from build123d import *

# Parameters (mm, degrees)
F1_DEPTH       = 120.65
F2_R           = 1.524
F4_D           = 20.6375
F4_CBORE_D     = 30.1752
F4_CBORE_DEPTH = 28.448
F5_W           = 63.5
F5_H           = 241.3
F6_DEPTH       = 6.35
F8_D           = 13.49248
F8_DEPTH       = 41.2172727273
F8_TIP         = 4.0535499425


# Not quite as in the source:
# - a length typed as a fraction of an inch, garbled in the dataset ("3 / 203.2 mm" for 3/8 in), is restored


with BuildPart() as f1:
    # F0 (on Top) → F1 (new body, symmetric)
    with BuildSketch(Plane.XY):
        Polygon((82.55, 44.45), (-82.55, 44.45), (-82.55, 31.75), (-44.45, 31.75), (-44.45, -31.75), (-82.55, -31.75), (-82.55, -44.45), (82.55, -44.45), align=None)
    extrude(amount=F1_DEPTH, both=True)

    # F2
    f2_edges = [f1.edges().sort_by_distance(p)[0] for p in [
        (-44.45, 31.75, 0),
        (-44.45, -31.75, 0),
    ]]
    fillet(f2_edges, radius=F2_R)

    # F4 (through all)
    with Locations(Plane.YZ.offset(82.55)):
        with Locations((0, 63.5), (0, -63.5)):
            CounterBoreHole(F4_D / 2, F4_CBORE_D / 2, F4_CBORE_DEPTH)

    # F5 (on face) → F6 (cut)
    with BuildSketch(Plane.XZ.offset(44.45)):
        with Locations((50.8, 0)):
            Rectangle(F5_W, F5_H)
    extrude(amount=-F6_DEPTH, mode=Mode.SUBTRACT)

    # F8
    with Locations(Plane.XZ.offset(38.1)):
        with Locations((50.8, 95.25), (50.8, 0), (50.8, -95.25)):
            Hole(F8_D / 2, depth=F8_DEPTH)
            with Locations((0, 0, -(F8_DEPTH + F8_TIP / 2))):  # 118° drill point
                Cone(0, F8_D / 2, F8_TIP, mode=Mode.SUBTRACT)


solid = f1.part
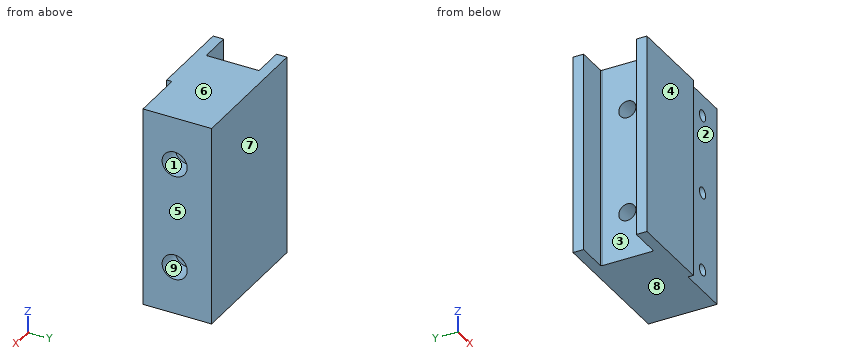
Could you check a few things on this model? Use its own coordinates, in mm. Face numbers are marked on the shaded views. A direction names the side the tool comes from. Round coordinates to 2 decimals unless told otherwise and drop trailing zeros. Order: outer loops, then holes, each group sorted by start corner. A loop starts at its lowest first (then second) coordinate and runs counter-clockwise, first axis right, second up.
(1) Imagine slicing it at A-A (y = 0). Write out the boundary of the cut face in (x, z), plus the area to 3 significant figures.
Response values:
outline: (-44.45, -120.65) - (82.55, -120.65) - (82.55, -78.59) - (54.1, -78.59) - (54.1, -73.82) - (-44.45, -73.82) - close; (-44.45, -53.18) - (54.1, -53.18) - (54.1, -48.41) - (82.55, -48.41) - (82.55, 48.41) - (54.1, 48.41) - (54.1, 53.18) - (-44.45, 53.18) - close; (-44.45, 73.82) - (54.1, 73.82) - (54.1, 78.59) - (82.55, 78.59) - (82.55, 120.65) - (-44.45, 120.65) - close; hole circle Ø13.49 at (50.8, -95.25); hole circle Ø13.49 at (50.8, 0); hole circle Ø13.49 at (50.8, 95.25)
area: 24,400 mm2
(2) I'm going to push flat-ended pins straight in: pin 1 (9 mm diameter, centred on y = 5.5, z = -59, fed in from +X); pin 2 (3 mm diameter, centred on y = -14.5, z = -48.5, fed in from -X); pin 3 (8 mm diameter, centred on x = 50.8, z = 95.25, fed in from -Y); pin 4 (24 mm diameter, centred on y = -2, z = 71, fed in from +X). Where does each tip first touch, or does it pass through?
Response values:
pin 1: stops at x = 54.1
pin 2: stops at x = -44.45
pin 3: stops at y = 4.77
pin 4: stops at x = 82.55
(3) Which directions (+Z, -Z, +X, -X, +Y, -Y) give clear straight access to the entire face, cutting with the end or side of a thin tool? Please do the marked faces 1, 2, 3, 4 and 5.
Response values:
face 1: +X
face 2: +Z, -Z, +X, -Y
face 3: +Z, -Z, -X
face 4: +Z, -Z, +X, -X, -Y
face 5: +Z, -Z, +X, +Y, -Y
(4) Please list where these lines run through material, in increasing order: line 1 along Z through (x, y) = (68, 0); line 2 along Z through (x, y) = (32, 0); line 3 along Z through (x, y) = (50.8, -24.5).
Response values:
line 1: z = -120.65 to -78.59, -48.41 to 48.41, 78.59 to 120.65
line 2: z = -120.65 to -73.82, -53.18 to 53.18, 73.82 to 120.65
line 3: z = -120.65 to -102, -88.5 to -6.75, 6.75 to 88.5, 102 to 120.65
(5) Imagine slicing it at B-B (x = -54). Write out the boundary of the cut face in (y, z), plus the area to 3 significant figures.
Response values:
outline: (-44.45, -120.65) - (-31.75, -120.65) - (-31.75, 120.65) - (-44.45, 120.65) - close; (31.75, -120.65) - (44.45, -120.65) - (44.45, 120.65) - (31.75, 120.65) - close
area: 6,130 mm2
(6) Imagine slicing it at D-D (x = -0.5). Write out the boundary of the cut face in (y, z).
Response values:
outline: (-44.45, -120.65) - (44.45, -120.65) - (44.45, 120.65) - (-44.45, 120.65) - close; hole circle Ø20.64 at (0, -63.5); hole circle Ø20.64 at (0, 63.5)
(7) Imagine slicing it at C-C (z = 63.5). Write out the boundary of the cut face in (x, y), plus the area to 3 significant figures.
Response values:
outline: (-82.55, -44.45) - (19.05, -44.45) - (19.05, -38.1) - (82.55, -38.1) - (82.55, -15.09) - (54.1, -15.09) - (54.1, -10.32) - (-44.45, -10.32) - (-44.45, -30.23) arc R1.52 cw to (-45.97, -31.75) - (-82.55, -31.75) - close; (-82.55, 31.75) - (-45.97, 31.75) arc R1.52 cw to (-44.45, 30.23) - (-44.45, 10.32) - (54.1, 10.32) - (54.1, 15.09) - (82.55, 15.09) - (82.55, 44.45) - (-82.55, 44.45) - close
area: 8,960 mm2
(8) If we mould it in two halves opening along Z, with no side actions, what happens to the marked faces 6, 7, 8 and 9? For each: released by +Z, released by -Z, zero draft, split by the parting line, or undercut.
Response values:
face 6: released by +Z
face 7: zero draft
face 8: released by -Z
face 9: undercut
